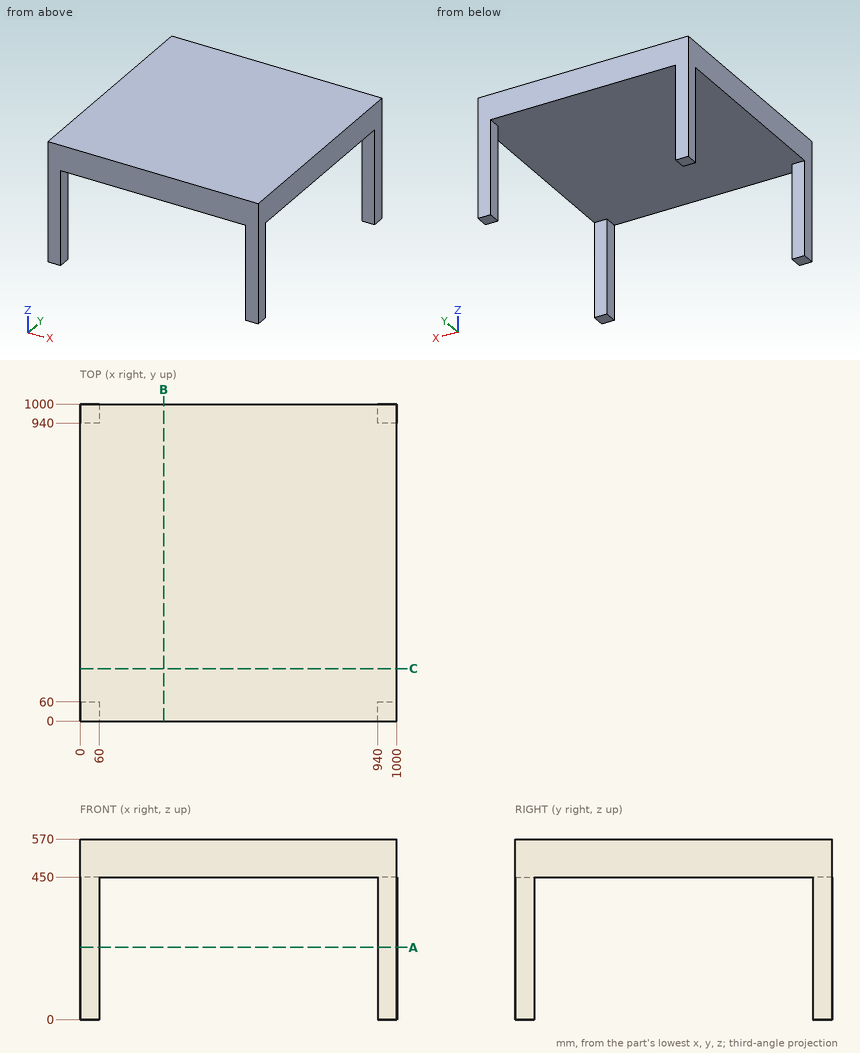
Here's the drawing with two shaded views (mm, measured from the low corner). I have some questions. Round coordinates to 2 decimals unless told otherwise and drop trailing zeros. Loops run counter-clockwise (first coordinate to the right, second up) from the corner with the lowest first, then second, coordinate; pieces in that order, holes last. Notation, with made-up numbers: (1.25, 36.25) -> (51.25, 36.25) arc R26 ccw to (51.25, 52.25) -> close; hole circle Ø2 at (58.5, 2). An arc over 180 degrees is marked (long way). Answer as CSV lines item,"result". Start each with the question number.
1. Imagine slicing it at A-A on z = 228. Write out the boundary of the cut face in (x, y).
2. I need wall thicknesses on probe 1 along Z at (x, y) = (356, 810). Which ranges of the line are inside material? Lowest first, please. Write a range as from..to.
3. I'm going to push a flat-ended pin straight in: P1, Ø10, axis at x = 644, y = 752, coming from the -Z side. Where does the tip first touch, or does it pass through?
4. Imagine slicing it at B-B on x = 264. Write out the boundary of the cut face in (y, z), plus the area to 3 significant figures.
Solution:
1,outline,"(0, 0) -> (60, 0) -> (60, 60) -> (0, 60) -> close; (0, 940) -> (60, 940) -> (60, 1000) -> (0, 1000) -> close; (940, 0) -> (1000, 0) -> (1000, 60) -> (940, 60) -> close; (940, 940) -> (1000, 940) -> (1000, 1000) -> (940, 1000) -> close"
2,probe 1,"450..570"
3,P1,"z = 450"
4,outline,"(0, 450) -> (1000, 450) -> (1000, 570) -> (0, 570) -> close"
4,area,"120,000 mm²"
